Here's the drawing with two shaded views (mm, measured from the low corner). I have some questions. A direction names the side the tool comes from. Round coordinates to 2 decimals unless told otherwise and drop trailing zeros. Loops run counter-clockwise (first coordinate to the right, second up) from the corner with the lowest first, then second, coordinate; pieces in that order, holes last.
(1) Which directions (+Z, -Z, +X, -X, +Y, -Y) give clear straight access to the entire face, cutting with the end or side of a thin tool? Please do the marked faces 1 and 2.
(2) I want a section at D-D on x = 2.75. Write out the boundary of the cut face in (y, z).
(3) I want a section at B-B on z = 9.8. Write out the boundary of the cut face in (x, y).
(4) I want a section at C-C on y = 42.2. Write out the boundary of the cut face in (x, z).
(5) If I drill on line 1 along Y through (x, z) = (7.9, 51.15); line 2 along Z through (x, y) = (7.9, 1.55); line 3 along Z through (x, y) = (4.75, 21), over which ranges is the centre line in solid material (lowest first)?
(6) I want a section at A-A on x = 7.9. Write out the boundary of the cut face in (y, z), plus the area to 3 significant figures.
(7) Will these pins go through, and if not, where does the flat tip stop? pin 1 Ø8 at (x, y) = (13, 10) entering from -Z; pin 2 Ø1.5 at (x, z) = (5.5, 30.5) entering from +Y; pin 3 Ø3.5 at (x, z) = (7.9, 9.8) entering from +Y.
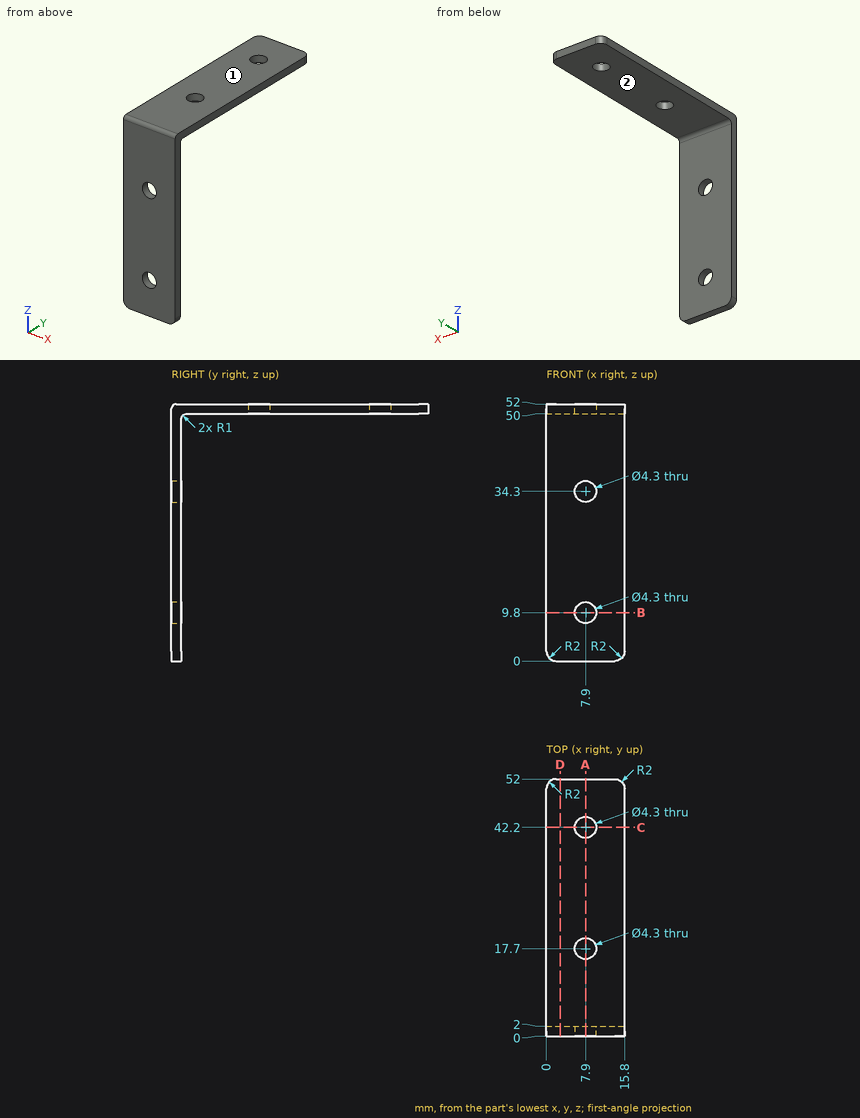
Filled sheet:
1. face 1: +Z, +X, -X, +Y, -Y
1. face 2: -Z, +X, -X, +Y
2. outline: (0, 0) - (2, 0) - (2, 49) arc R1 cw to (3, 50) - (52, 50) - (52, 52) - (1, 52) arc R1 ccw to (0, 51) - close
3. outline: (0, 0) - (5.75, 0) - (5.75, 2) - (0, 2) - close; (10.05, 0) - (15.8, 0) - (15.8, 2) - (10.05, 2) - close
4. outline: (0, 50) - (5.75, 50) - (5.75, 52) - (0, 52) - close; (10.05, 50) - (15.8, 50) - (15.8, 52) - (10.05, 52) - close
5. line 1: y = 0.01 to 15.55, 19.85 to 40.05, 44.35 to 52
5. line 2: z = 0 to 7.65, 11.95 to 32.15, 36.45 to 52
5. line 3: z = 50 to 52
6. outline: (0, 0) - (2, 0) - (2, 7.65) - (0, 7.65) - close; (0, 11.95) - (2, 11.95) - (2, 32.15) - (0, 32.15) - close; (0, 36.45) - (2, 36.45) - (2, 49) arc R1 cw to (3, 50) - (15.55, 50) - (15.55, 52) - (1, 52) arc R1 ccw to (0, 51) - close; (19.85, 50) - (40.05, 50) - (40.05, 52) - (19.85, 52) - close; (44.35, 50) - (52, 50) - (52, 52) - (44.35, 52) - close
6. area: 170 mm2
7. pin 1: stops at z = 50
7. pin 2: stops at y = 2
7. pin 3: passes through
